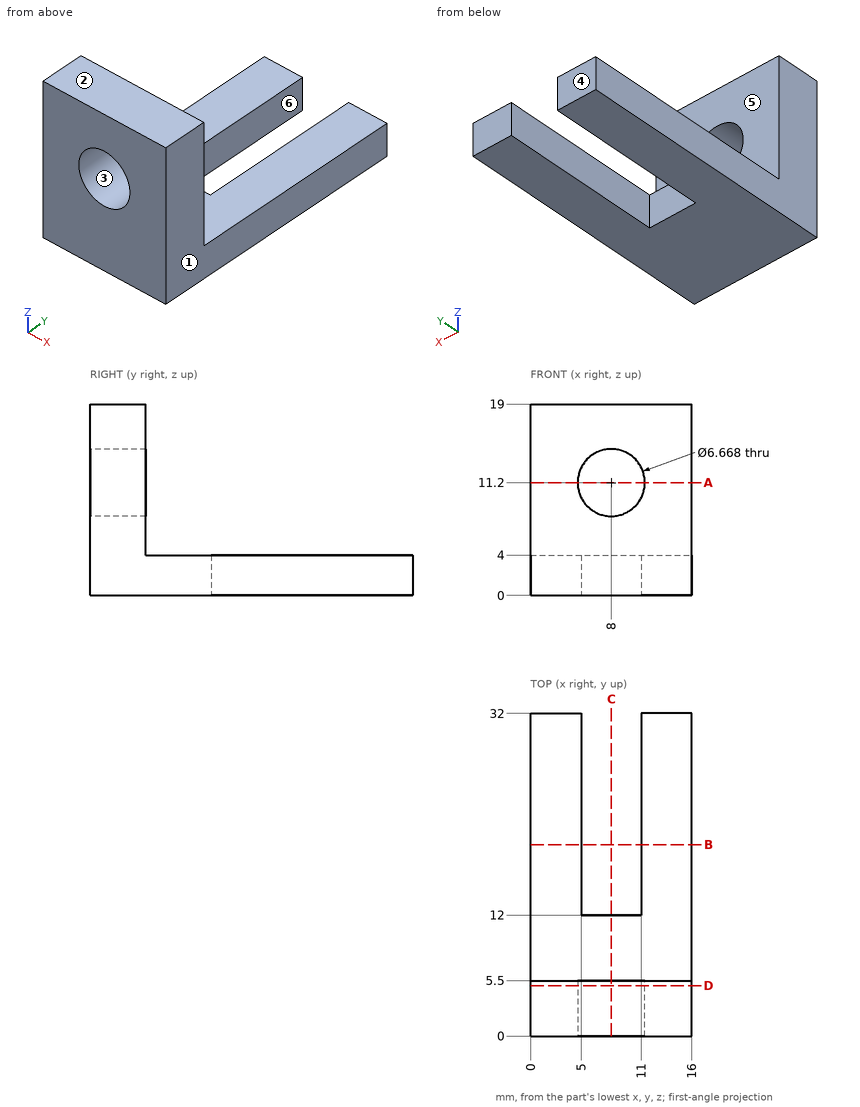
The drawing under review shows one solid part. Ordinate dimensions are in mm from its lowest x, y, z. A direction names the side the tool comes from. Round coordinates to 2 decimals unless told otherwise and drop trailing zeros. Write each loop counter-clockwise with the first axis right and the second up, starting at its lowest first coordinate (ties: lowest second). Pieces come first, ordered by that corner, then holes.
(1) We need section B-B on y = 19. Give the boundary of the cut face in (x, z).
(2) Mouldability with a two-part tool opening along X and no side actions: class the marked faces 1, 2 and 3 as +X half, -X half, draft (parallel to the pull), parting line (faces both ways), or undercut.
(3) Wall thickness on L1, parallel to Z at x = 8, y = 2.8; L2, parallel to Z at x = 13.5, y = 24; L3, parallel to Y at x = 11.5, z = 16.25: over which ranges is each line inside the solid? List them lowest first.
(4) Machinability: for the marked faces 4, 5 and 6, which of the approach directions +Z, -Z, +X, -X, +Y, -Y give a long, thin tool a straight path to every point of the face, cutting with its end or side? Answer none if there is none.
(5) We need section A-A on z = 11.2. Give the boundary of the cut face in (x, y).
(6) We need section D-D on y = 5. Give the boundary of the cut face in (x, z).
(7) We need section C-C on x = 8. Give the boundary of the cut face in (y, z).
(8) Insertion check: pin 1 (2 mm diameter, centred on x = 6.5, z = 3, fed in from +Y); pin 2 (8 mm diameter, centred on x = 12.5, z = 17, fed in from +Y); pin 3 (1 mm diameter, centred on x = 7, y = 10, fed in from +Z). Each pin has a flat end and moves straight along its axis. Give the tip position at first contact, or say it passes through.
Findings below:
1. outline: (0, 0) - (5, 0) - (5, 4) - (0, 4) - close; (11, 0) - (16, 0) - (16, 4) - (11, 4) - close
2. face 1: +X half
2. face 2: draft
2. face 3: undercut
3. L1: z = 0 to 7.87, 14.53 to 19
3. L2: z = 0 to 4
3. L3: y = 0 to 5.5
4. face 4: +Z, -Z, +X, -X, +Y
4. face 5: +Z, +X, -X, +Y
4. face 6: +Z, -Z, +Y
5. outline: (0, 0) - (4.67, 0) - (4.67, 5.5) - (0, 5.5) - close; (11.33, 0) - (16, 0) - (16, 5.5) - (11.33, 5.5) - close
6. outline: (0, 0) - (16, 0) - (16, 19) - (0, 19) - close; hole circle Ø6.67 at (8, 11.2)
7. outline: (0, 0) - (12, 0) - (12, 4) - (5.5, 4) - (5.5, 7.87) - (0, 7.87) - close; (0, 14.53) - (5.5, 14.53) - (5.5, 19) - (0, 19) - close
8. pin 1: stops at y = 12
8. pin 2: stops at y = 5.5
8. pin 3: stops at z = 4
